Can you work these out from the model? Positions are in its coordinate system, mm. Round coordinates to 2 decimals unless told otherwise and drop trailing zeros. Write each loop counter-clockwise with the first axis right and the second up, starting at its lowest first coordinate (ties: lowest second). Pieces come first, ordered by that corner, then holes.
Q1. I'm going to push flat-ended pins straight in: pin 1 Ø1 at (y, z) = (-71.5, 5) entering from +X; pin 2 Ø4 at (x, z) = (-53, 6.5) entering from -Y; pin 3 Ø5 at (x, z) = (-80, 2.5) entering from -Y. Where does each tip first touch, or does it pass through?
Q2. Please list where these lines run through material, in increasing order: line 1 along X through (y, z) = (-2.5, 10.25); line 2 along Y through (x, z) = (-25, 10.5); line 3 along X through (y, z) = (4.5, 3.5).
Q3. If we section it at A-A (x = 0): Please give me the cut outline in (y, z), plus the area to 3 significant figures.
Q4. If we section it at C-C (z = 7.75): Give the number of separate pieces and of enclosed holes in the cut face, plus the area to 3 significant figures.
Q5. We'd pull the mould along X, two halves only. Please class faces 1 (the cylindrical face through (-1.915, 82.881, 7.605)), 2 (the flat face through (-2, 2, 15)), 3 (the cylindrical face through (86.941, 85.932, 1.426)): +X half, -X half, draft (parallel to the pull), parting line (faces both ways), or undercut.
from build123d import *

# Parameters (mm, degrees)
F0_W            = 250
F0_H            = 250
F1_DEPTH        = 15
F3_R            = 5
F4_DEPTH        = 15.001
F4_COPIES_COUNT = 7
F4_COPIES_ANGLE = 270
F6_R            = 7.5
F7_DEPTH        = 15.001
F8_SIZE         = 75
F9_R            = 5


# Not quite as in the source:
# - a pattern or mirror of a feature is missing from the dataset's text; its kind, count and spacing are read off the source's solid


with BuildPart() as f1:
    # F0 (on Top) → F1 (new body)
    with BuildSketch(Plane.XY):
        Rectangle(F0_W, F0_H)
    extrude(amount=F1_DEPTH)

    # F3 (on face) → F4 (cut, through all)
    with BuildSketch(Plane.XY.offset(15)):
        with Locations((-87.5, 0)):
            Circle(F3_R)
    f4 = extrude(amount=-F4_DEPTH, mode=Mode.SUBTRACT)

    # F4_copies: F4 ×7 about axis
    f4_copies_axis = Axis((0, 0, 0), (0, 0, -1))
    for i in range(1, F4_COPIES_COUNT):
        add(f4.rotate(f4_copies_axis, i * F4_COPIES_ANGLE / (F4_COPIES_COUNT - 1)), mode=Mode.SUBTRACT)

    # F6 (on face) → F7 (cut, through all)
    with BuildSketch(Plane.XY.offset(15)):
        with Locations((-61.8718433538, -61.8718433538)):
            Circle(F6_R)
    extrude(amount=-F7_DEPTH, mode=Mode.SUBTRACT)

    # F8
    f8_edges = [f1.edges().sort_by_distance(p)[0] for p in [
        (-125, 125, 7.5),
        (-125, -125, 7.5),
        (125, -125, 7.5),
        (125, 125, 7.5),
    ]]
    chamfer(f8_edges, length=F8_SIZE)

    # F9
    f9_edges = [f1.edges().sort_by_distance(p)[0] for p in [
        (-125, 0, 15),
        (-125, 0, 0),
        (-125, 50, 7.5),
        (-125, -50, 7.5),
        (-87.5, -87.5, 0),
        (-50, -125, 7.5),
        (-87.5, -87.5, 15),
        (0, -125, 0),
        (50, -125, 7.5),
        (0, -125, 15),
        (87.5, -87.5, 0),
        (125, -50, 7.5),
        (87.5, -87.5, 15),
        (125, 0, 0),
        (125, 50, 7.5),
        (125, 0, 15),
        (87.5, 87.5, 0),
        (50, 125, 7.5),
        (87.5, 87.5, 15),
        (0, 125, 0),
        (-50, 125, 7.5),
        (0, 125, 15),
        (-87.5, 87.5, 0),
        (-87.5, 87.5, 15),
    ]]
    fillet(f9_edges, radius=F9_R)


solid = f1.part
A:
1. pin 1: stops at x = 104
1. pin 2: stops at y = -123.95
1. pin 3: stops at y = -96.97
2. line 1: x = -124.99 to -91.83, -83.17 to 83.17, 91.83 to 124.99
2. line 2: y = -124.97 to 124.97
2. line 3: x = -124.77 to -89.68, -85.32 to 85.32, 89.68 to 124.77
3. outline: (-125, 5) arc R5 ccw to (-120, 0) - (-92.5, 0) - (-92.5, 15) - (-120, 15) arc R5 ccw to (-125, 10) - close; (-82.5, 0) - (82.5, 0) - (82.5, 15) - (-82.5, 15) - close; (92.5, 0) - (120, 0) arc R5 ccw to (125, 5) - (125, 10) arc R5 ccw to (120, 15) - (92.5, 15) - close
3. area: 3,430 mm2
4. separate pieces: 1
4. enclosed holes: 8
4. area: 50,500 mm2
5. face 1: undercut
5. face 2: draft
5. face 3: +X half
